```python
from build123d import *

# Parameters (mm, degrees)
SKETCH_1_W               = 380
SKETCH_1_H               = 148
EXTRUDE_1_DEPTH          = 10
SKETCH_2_W               = 260
SKETCH_2_H               = 56
EXTRUDE_2_DEPTH          = 325
SKETCH_3_W               = 280
SKETCH_3_H               = 148
EXTRUDE_3_DEPTH          = 10
SKETCH_4_R               = 120
CUT_EXTRUDE_1_DEPTH      = 526.327516888
SKETCH_5_R               = 120
SKETCH_5_R_2             = 80
EXTRUDE_4_DEPTH          = 148
SKETCH_6_W               = 10
SKETCH_6_H               = 36
EXTRUDE_5_DEPTH          = 50
SKETCH_7_W               = 50
SKETCH_7_H               = 10
EXTRUDE_6_DEPTH          = 50
CUT_EXTRUDE_2_DEPTH      = 526.327516888
SKETCH_9_R               = 80
SKETCH_9_R_2             = 65
EXTRUDE_7_DEPTH          = 14
SKETCH_10_R              = 65
SKETCH_10_R_2            = 45
EXTRUDE_8_DEPTH          = 6
EXTRUDE_START            = 10
SKETCH_11_R              = 120
SKETCH_11_R_2            = 45
EXTRUDE_9_DEPTH          = 10
EXTRUDE_START_2          = -14
SKETCH_12_R              = 80
SKETCH_12_R_2            = 65
EXTRUDE_10_DEPTH         = 14
EXTRUDE_START_3          = -5
SKETCH_13_R              = 65
EXTRUDE_11_DEPTH         = 5
SKETCH_14_R              = 120
EXTRUDE_12_DEPTH         = 10
SKETCH_15_R              = 8.5
CUT_EXTRUDE_3_DEPTH      = 10
SKETCH_16_R              = 5
CUT_EXTRUDE_4_DEPTH      = 25
CUT_EXTRUDE_START        = -25
SKETCH_17_R              = 5
CUT_EXTRUDE_5_DEPTH      = 25
PATTERN_CIRCULAR_1_COUNT = 8


with BuildPart() as part:
    # Sketch 1 → Extrude 1 (new body)
    with BuildSketch(Plane(origin=(0, 0, 0), x_dir=(1, 0, 0), z_dir=(0, 1, 0))):
        with Locations((190, 74)):
            Rectangle(SKETCH_1_W, SKETCH_1_H)
    extrude(amount=EXTRUDE_1_DEPTH)

    # Sketch 2 → Extrude 2 (add)
    with BuildSketch(Plane(origin=(0, 10, 0), x_dir=(1, 0, 0), z_dir=(0, 1, 0))):
        Polygon((50, 148), (60, 148), (60, 112), (320, 112), (320, 148), (330, 148), (330, 0), (320, 0), (320, 36), (60, 36), (60, 0), (50, 0), align=None)
        with Locations((190, 74)):
            Rectangle(SKETCH_2_W, SKETCH_2_H, mode=Mode.SUBTRACT)
    extrude(amount=EXTRUDE_2_DEPTH)

    # Sketch 3 → Extrude 3 (add)
    with BuildSketch(Plane(origin=(0, 335, 0), x_dir=(1, 0, 0), z_dir=(0, 1, 0))):
        with Locations((190, 74)):
            Rectangle(SKETCH_3_W, SKETCH_3_H)
    extrude(amount=EXTRUDE_3_DEPTH)

    # Sketch 4 → Cut-Extrude 1 (cut, through all)
    with BuildSketch(Plane.XY.offset(-36)):
        with Locations((190, 175)):
            Circle(SKETCH_4_R)
    extrude(amount=-CUT_EXTRUDE_1_DEPTH, mode=Mode.SUBTRACT)

    # Sketch 5 → Extrude 4 (add)
    with BuildSketch(Plane.XY):
        with Locations((190, 175)):
            Circle(SKETCH_5_R)
        with Locations((190, 175)):
            Circle(SKETCH_5_R_2, mode=Mode.SUBTRACT)
    extrude(amount=-EXTRUDE_4_DEPTH)

    # Sketch 6 → Extrude 5 (add)
    with BuildSketch(Plane(origin=(0, 10, 0), x_dir=(1, 0, 0), z_dir=(0, 1, 0))):
        with Locations((145, 18)):
            Rectangle(SKETCH_6_W, SKETCH_6_H)
        with Locations((235, 18)):
            Rectangle(SKETCH_6_W, SKETCH_6_H)
        with Locations((235, 130)):
            Rectangle(SKETCH_6_W, SKETCH_6_H)
        with Locations((145, 130)):
            Rectangle(SKETCH_6_W, SKETCH_6_H)
    extrude(amount=EXTRUDE_5_DEPTH)

    # Sketch 7 → Extrude 6 (add)
    with BuildSketch(Plane(origin=(0, 10, 0), x_dir=(1, 0, 0), z_dir=(0, 1, 0))):
        with Locations((355, 41)):
            Rectangle(SKETCH_7_W, SKETCH_7_H)
        with Locations((355, 107)):
            Rectangle(SKETCH_7_W, SKETCH_7_H)
        with Locations((25, 107)):
            Rectangle(SKETCH_7_W, SKETCH_7_H)
        with Locations((25, 41)):
            Rectangle(SKETCH_7_W, SKETCH_7_H)
    extrude(amount=EXTRUDE_6_DEPTH)

    # Sketch 8 → Cut-Extrude 2 (cut, through all)
    with BuildSketch(Plane(origin=(0, 0, -112), x_dir=(-1, 0, 0), z_dir=(0, 0, -1))):
        Polygon((-380, 60), (-350, 60), (-380, 30), align=None)
        Polygon((0, 60), (-30, 60), (0, 30), align=None)
    extrude(amount=-CUT_EXTRUDE_2_DEPTH, mode=Mode.SUBTRACT)



with BuildPart() as body_2:
    # Sketch 9 → Extrude 7 (new body)
    with BuildSketch(Plane.XY):
        with Locations((190, 175)):
            Circle(SKETCH_9_R)
        with Locations((190, 175)):
            Circle(SKETCH_9_R_2, mode=Mode.SUBTRACT)
    extrude(amount=-EXTRUDE_7_DEPTH)


with BuildPart() as part_1:
    add(part.part)

    add(body_2.part)  # Extrude 8 merges body 2
    # Sketch 10 → Extrude 8 (add)
    with BuildSketch(Plane.XY):
        with Locations((190, 175)):
            Circle(SKETCH_10_R)
        with Locations((190, 175)):
            Circle(SKETCH_10_R_2, mode=Mode.SUBTRACT)
    extrude(amount=-EXTRUDE_8_DEPTH)

    # Sketch 11 → Extrude 9 (add)
    with BuildSketch(Plane.XY.offset(EXTRUDE_START)):
        with Locations((190, 175)):
            Circle(SKETCH_11_R)
        with Locations((190, 175)):
            Circle(SKETCH_11_R_2, mode=Mode.SUBTRACT)
    extrude(amount=-EXTRUDE_9_DEPTH)

    # Sketch 12 → Extrude 10 (add)
    with BuildSketch(Plane(origin=(0, 0, -148), x_dir=(-1, 0, 0), z_dir=(0, 0, -1)).offset(EXTRUDE_START_2)):
        with Locations(Location((-190, 175, 0), (0, 0, 180))):
            Circle(SKETCH_12_R)
        with Locations(Location((-190, 175, 0), (0, 0, 180))):
            Circle(SKETCH_12_R_2, mode=Mode.SUBTRACT)
    extrude(amount=EXTRUDE_10_DEPTH)

    # Sketch 13 → Extrude 11 (add)
    with BuildSketch(Plane(origin=(0, 0, -148), x_dir=(-1, 0, 0), z_dir=(0, 0, -1)).offset(EXTRUDE_START_3)):
        with Locations((-190, 175)):
            Circle(SKETCH_13_R)
    extrude(amount=EXTRUDE_11_DEPTH)

    # Sketch 14 → Extrude 12 (add)
    with BuildSketch(Plane(origin=(0, 0, -148), x_dir=(-1, 0, 0), z_dir=(0, 0, -1))):
        with Locations(Location((-190, 175, 0), (0, 0, 180))):
            Circle(SKETCH_14_R)
    extrude(amount=EXTRUDE_12_DEPTH)

    # Sketch 15 → Cut-Extrude 3 (cut)
    with BuildSketch(Plane.XZ):
        with Locations(Location((25, -129, 0), (0, 0, 270))):
            Circle(SKETCH_15_R)
        with Locations(Location((25, -74, 0), (0, 0, 270))):
            Circle(SKETCH_15_R)
        with Locations(Location((25, -19, 0), (0, 0, 270))):
            Circle(SKETCH_15_R)
        with Locations(Location((190, -129, 0), (0, 0, 270))):
            Circle(SKETCH_15_R)
        with Locations(Location((100, -129, 0), (0, 0, 270))):
            Circle(SKETCH_15_R)
        with Locations(Location((280, -129, 0), (0, 0, 270))):
            Circle(SKETCH_15_R)
        with Locations(Location((355, -74, 0), (0, 0, 270))):
            Circle(SKETCH_15_R)
        with Locations(Location((355, -129, 0), (0, 0, 270))):
            Circle(SKETCH_15_R)
        with Locations(Location((355, -19, 0), (0, 0, 270))):
            Circle(SKETCH_15_R)
    extrude(amount=-CUT_EXTRUDE_3_DEPTH, mode=Mode.SUBTRACT)

    # Sketch 16 → Cut-Extrude 4 (cut)
    with BuildSketch(Plane.XY.offset(10)):
        with Locations((190, 275)):
            Circle(SKETCH_16_R)
    cut_extrude_4 = extrude(amount=-CUT_EXTRUDE_4_DEPTH, mode=Mode.SUBTRACT)

    # Sketch 17 → Cut-Extrude 5 (cut)
    with BuildSketch(Plane(origin=(0, 0, -158), x_dir=(-1, 0, 0), z_dir=(0, 0, -1)).offset(CUT_EXTRUDE_START)):
        with Locations(Location((-190, 275, 0), (0, 0, 180))):
            Circle(SKETCH_17_R)
    cut_extrude_5 = extrude(amount=CUT_EXTRUDE_5_DEPTH, mode=Mode.SUBTRACT)

    # Pattern Circular 1: Cut-Extrude 4, Cut-Extrude 5 ×8 about axis
    pattern_circular_1_axis = Axis((190, 175, 0), (0, 0, 1))
    add([cut_extrude_4.rotate(pattern_circular_1_axis, i * 360 / PATTERN_CIRCULAR_1_COUNT) for i in range(1, PATTERN_CIRCULAR_1_COUNT)], mode=Mode.SUBTRACT)
    add([cut_extrude_5.rotate(pattern_circular_1_axis, i * 360 / PATTERN_CIRCULAR_1_COUNT) for i in range(1, PATTERN_CIRCULAR_1_COUNT)], mode=Mode.SUBTRACT)


solid = part_1.part
```
Could you check a few things on this model? Use its own coordinates, in mm. A direction names the side the tool comes from. Give positions to 0.01 mm unless a question says otherwise; leave off trailing zeros. Loops run counter-clockwise (first coordinate to the right, second up) from the corner with the lowest first, then second, coordinate; pieces in that order, holes last. Notation, with made-up numbers: (-14, 8.5) -> (40, 8.5) arc R20 ccw to (40, 36.5) -> close; hole circle Ø10 at (-24.5, -11.75). An arc over 180 degrees is marked (long way). Put each result on its own line as item: value.
(1) I'm going to push flat-ended pins straight in: pin 1 Ø25 at (x, y) = (19.5, 35.5) entering from +Z; pin 2 Ø12 at (y, z) = (164, -26.5) entering from +X; pin 3 Ø10 at (y, z) = (183.5, -114.5) entering from -X. Where does each tip first touch, or does it pass through?
Computed:
pin 1: z = -36
pin 2: x = 330
pin 3: x = 50
(2) Please list where these lines run through material, in increasing order: probe 1 along X at (y, z) = (45, -25); probe 2 along Y at (x, z) = (190, 2.75); probe 3 along X at (y, z) = (200, -127.5). Write a range as [from, to].
Computed:
probe 1: [50, 60], [140, 150], [230, 240], [320, 330]
probe 2: [55, 70], [80, 130], [220, 270], [280, 295]
probe 3: [50, 60], [72.63, 114.01], [265.99, 307.37], [320, 330]
(3) For faces 1 (the face through (349, 29, -102)), 2 (the face through (30, 29, -46)), 3 (the face through (140, 35, -18)), 4 (the face through (279, 10, -138)), which set-ups out of +Z, -Z, +X, -X, +Y, -Y let a thin tool reach every point of the face, with its end or its side?
Computed:
face 1: +X, +Y
face 2: -X, +Y
face 3: +Z
face 4: -Z
(4) Imagine slicing it at B-B on y = 317. Write out the boundary of the cut face in (x, z), plus the area to 3 significant figures.
Computed:
outline: (50, -148) -> (60, -148) -> (60, -112) -> (320, -112) -> (320, -148) -> (330, -148) -> (330, 0) -> (320, 0) -> (320, -36) -> (60, -36) -> (60, 0) -> (50, 0) -> close; hole (60, -102) -> (320, -102) -> (320, -46) -> (60, -46) -> close
area: 8,160 mm^2
(5) Imagine slicing it at C-C on x = 190. State how many separate pieces and enclosed holes the cut face has, plus the area to 3 significant figures.
Computed:
separate pieces: 2
enclosed holes: 2
area: 21,000 mm^2
(6) Thinking about a two-plate mould opening in Y: for faces 5 (the face through (363.428, 4.93, -127.893)), 6 (the face through (365, 45, -107)), 7 (the face through (120.79, 109.06, -2.32)), which applies, pulls with the +Y half, pulls with the -Y half, needs draft (parallel to the pull), parting line crosses it, or undercut?
Computed:
face 5: needs draft
face 6: pulls with the +Y half
face 7: undercut
(7) Imagine slicing it at A-A on z = -74. Write out the boundary of the cut face in (x, y), plus the area to 3 significant figures.
Computed:
outline: (0, 0) -> (16.5, 0) -> (16.5, 10) -> (0, 10) -> close; (33.5, 0) -> (346.5, 0) -> (346.5, 10) -> (330, 10) -> (330, 345) -> (50, 345) -> (50, 10) -> (33.5, 10) -> close; circle Ø240 at (190, 175); (363.5, 0) -> (380, 0) -> (380, 10) -> (363.5, 10) -> close; hole (60, 10) -> (320, 10) -> (320, 335) -> (60, 335) -> close; hole circle Ø160 at (190, 175)
area: 37,900 mm^2
